Here's how the part is built. I have some questions about the finished solid (model axes, mm). A direction names the side the tool comes from. Round coordinates to 2 decimals unless told otherwise and drop trailing zeros. Write each loop counter-clockwise with the first axis right and the second up, starting at its lowest first coordinate (ties: lowest second). Pieces come first, ordered by that corner, then holes. Notation, with made-up numbers: (-13, 52) -> (18, 52) arc R20 cw to (18, 90) -> close; hole circle Ø2 at (56.25, 71.5). An arc over 180 degrees is marked (long way). Put each result on its own line as item: value. Start each with the question number.
1. Suppose I cut it at A-A (x = 14). Please give me the cut outline in (y, z).
2. Suppose I cut it at B-B (z = 1). Please give me the cut outline in (x, y), then the cut area to 3 significant figures.
3. Which directions (+Z, -Z, +X, -X, +Y, -Y) give clear straight access to the entire face, cutting with the end or side of a thin tool? Please do faces 1 (the face through (8, -11, 5)), 2 (the face through (0, 0, 0)).
4. I need wall thicknesses on probe 1 along Z at (x, y) = (-3, 15.5); probe 2 along Y at (x, z) = (0.5, 3.75); probe 3 along Y at (x, z) = (-4, 8). Which ranges of each line are inside material? Lowest first, please. Write a range as from..to.
5. Suppose I cut it at C-C (x = -14.5). Please give me the cut outline in (y, z), then the cut area to 3 significant figures.
6. For pin 1 (10 mm diameter, centred on x = 8, y = 11.5, fed in from +Z); pin 2 (1.5 mm diameter, centred on y = -0.5, z = 7, fed in from -X); pin 3 (2 mm diameter, centred on y = -12.5, z = 3, fed in from +X), each with a flat end and sliding along its axis, tell me the tip position at first contact or that it passes through.
```python
from build123d import *

# Parameters (mm, degrees)
F0_R     = 17.5
F1_DEPTH = 5
F2_R     = 12.5
F3_DEPTH = 5


# Not quite as in the source:
# - a fillet or chamfer that OpenCascade refuses, or shapes differently, is made with other operations: its cross-section is extruded or revolved along the edge and cut away or added


with BuildPart() as f1:
    # F0 (on Top) → F1 (new body)
    with BuildSketch(Plane.XY):
        Circle(F0_R)
    extrude(amount=F1_DEPTH)

    # F2 (on face) → F3 (join)
    with BuildSketch(Plane.XY.offset(5)):
        Circle(F2_R)
    extrude(amount=F3_DEPTH)

    # F4: fillet of radius 18 on 1 edges, made by hand

    # F4_s1 → F4_t2 (revolve, cut)
    with BuildSketch(Plane.XZ):
        with BuildLine():
            ThreePointArc((12.5, 5), (6.7583043345, 8.7032930885), (0.050100402, 10))
            Line((0.050100402, 10), (0.050100402, 10.36))
            Line((0.050100402, 10.36), (12.5, 10.36))
            Line((12.5, 10.36), (12.86, 10))
            ThreePointArc((12.86, 10), (12.86, 7.5), (12.748997992, 5.26))
            Line((12.748997992, 5.26), (12.5, 5))
        make_face()
    revolve(axis=Axis((0, 0, 10), (0, 0, 1)), mode=Mode.SUBTRACT)


solid = f1.part
```
Verdict:
1. outline: (-10.5, 0) -> (10.5, 0) -> (10.5, 5) -> (-10.5, 5) -> close
2. outline: circle Ø35 at (0, 0)
2. area: 962 mm^2
3. face 1: +Z
3. face 2: -Z, +X, -X, +Y, -Y
4. probe 1: z = 0..5
4. probe 2: y = -17.49..17.49
4. probe 3: y = -7.27..7.27
5. outline: (-9.8, 0) -> (9.8, 0) -> (9.8, 5) -> (-9.8, 5) -> close
5. area: 98.0 mm^2
6. pin 1: stops at z = 7.61
6. pin 2: stops at x = -11.04
6. pin 3: stops at x = 13.19
